Verification items for the finished model (mm, model axes). A direction names the side the tool comes from. Coordinates: 2 decimals unless noted, no trailing zeros. Write each loop counter-clockwise with the first axis right and the second up, starting at its lowest first coordinate (ties: lowest second). Pieces come first, ordered by that corner, then holes. Notation, with made-up numbers: (45.25, 66.5) -> (81.25, 66.5) arc R23 ccw to (81.25, 74.5) -> close; hole circle Ø8 at (57.25, 77.5). An arc over 180 degrees is marked (long way). Answer in a Markdown table with one row per item.
```python
from build123d import *

# Parameters (mm, degrees)
SKETCH_W        = 215
SKETCH_H        = 90
PAD_DEPTH       = 40
SKETCH001_W     = 200
SKETCH001_H     = 80
POCKET_DEPTH    = 10
SKETCH002_W     = 200
SKETCH002_H     = 13.845135
POCKET001_DEPTH = 10
POCKET002_DEPTH = 20
SKETCH004_W     = 40
SKETCH004_H     = 20
PAD001_DEPTH    = 40


with BuildPart() as part:
    # Sketch → Pad (new body)
    with BuildSketch(Plane.XY):
        Rectangle(SKETCH_W, SKETCH_H)
    extrude(amount=PAD_DEPTH)

    # Sketch001 (on Face6 of Pad) → Pocket (cut)
    with BuildSketch(Plane.XY.offset(40)):
        Rectangle(SKETCH001_W, SKETCH001_H)
    extrude(amount=-POCKET_DEPTH, mode=Mode.SUBTRACT)

    # Sketch002 (on Face5 of Pocket) → Pocket001 (cut)
    with BuildSketch(Plane.XY.offset(40)):
        with Locations((0.151818, -40.134584)):
            Rectangle(SKETCH002_W, SKETCH002_H)
    extrude(amount=-POCKET001_DEPTH, mode=Mode.SUBTRACT)

    # Sketch003 (on Face14 of Pocket001) → Pocket002 (cut)
    with BuildSketch(Plane.XY.offset(30)):
        with BuildLine():
            ThreePointArc((-50, 35), (-85, 0), (-50, -35))
            Line((-50, -35), (50, -35))
            ThreePointArc((50, -35), (85, 0), (50, 35))
            Line((50, 35), (-50, 35))
        make_face()
    extrude(amount=-POCKET002_DEPTH, mode=Mode.SUBTRACT)

    # Sketch004 (on Face6 of Pocket002) → Pad001 (join)
    with BuildSketch(Plane.XZ.offset(45)):
        with Locations((-87.5, 10)):
            Rectangle(SKETCH004_W, SKETCH004_H)
        with Locations((87.5, 10)):
            Rectangle(SKETCH004_W, SKETCH004_H)
    extrude(amount=PAD001_DEPTH)


solid = part.part
```
1. Section check C-C, the plane x = -5. Record the boundary of the cut face in (y, z).
Geometry says:
| item | result |
|---|---|
| outline | (-45, 0) -> (45, 0) -> (45, 40) -> (40, 40) -> (40, 30) -> (35, 30) -> (35, 10) -> (-35, 10) -> (-35, 30) -> (-45, 30) -> close |
2. Section check B-B, the plane z = 35. Record the boundary of the cut face in (x, y), plus the area to 3 significant figures.
Geometry says:
| item | result |
|---|---|
| outline | (-107.5, -45) -> (-99.85, -45) -> (-99.85, -40) -> (-100, -40) -> (-100, 40) -> (100, 40) -> (100, -33.21) -> (100.15, -33.21) -> (100.15, -45) -> (107.5, -45) -> (107.5, 45) -> (-107.5, 45) -> close |
| area | 2,350 mm^2 |
3. Tool access check on faces 1 (the flat face through (-1, -35, 20)), 2 (the flat face through (100.152, -39, 35)), 3 (the flat face through (87, -65, 20)), 4 (the flat face through (67.5, -65, 10)). Record the directions out of +Z, -Z, +X, -X, +Y, -Y that give a thin tool (end or side, any length) a straight path to the whole face; none if there is none.
Geometry says:
| item | result |
|---|---|
| face 1 | +Z |
| face 2 | +Z, -Y |
| face 3 | +Z, +X, -X, -Y |
| face 4 | +Z, -Z, -Y |
4. Depth check by flat-ended pin: P1, Ø6, axis at x = 11.5, z = 24.5, coming from the -Y side; P2, Ø8, axis at x = 7, z = 36, coming from the -Y side; P3, Ø4, axis at x = -48, y = -4, coming from the -Z side; P4, Ø3, axis at x = 67, y = 15, coming from the +Z side. Enter the tip coordinate at first touch or a pass-through.
Geometry says:
| item | result |
|---|---|
| P1 | y = -45 |
| P2 | y = 40 |
| P3 | z = 0 |
| P4 | z = 10 |
5. Thickness scan on line 1 (X direction, y = -46, z = 15.5); line 2 (X direction, y = -10.5, z = 37); line 3 (Y direction, x = -6, z = 25). Record the ranges inside material, lowest first. Write a range as from..to.
Geometry says:
| item | result |
|---|---|
| line 1 | -107.5..-67.5, 67.5..107.5 |
| line 2 | -107.5..-100, 100..107.5 |
| line 3 | -45..-35, 35..45 |
6. Mould release check, pull along X, two halves, no side actions. Record for faces 5 (the flat face through (-107.5, -5, 20)), 6 (the flat face through (-2, -5, 0)), 7 (the flat face through (-2, -45, 15)): released by +X, released by -X, zero draft, split by the parting line, or undercut.
Geometry says:
| item | result |
|---|---|
| face 5 | released by -X |
| face 6 | zero draft |
| face 7 | undercut |
7. Section check D-D, the plane z = 7.5. Record the boundary of the cut face in (x, y).
Geometry says:
| item | result |
|---|---|
| outline | (-107.5, -85) -> (-67.5, -85) -> (-67.5, -45) -> (67.5, -45) -> (67.5, -85) -> (107.5, -85) -> (107.5, 45) -> (-107.5, 45) -> close |
8. Section check A-A, the plane y = 0. Record the boundary of the cut face in (x, z).
Geometry says:
| item | result |
|---|---|
| outline | (-107.5, 0) -> (107.5, 0) -> (107.5, 40) -> (100, 40) -> (100, 30) -> (85, 30) -> (85, 10) -> (-85, 10) -> (-85, 30) -> (-100, 30) -> (-100, 40) -> (-107.5, 40) -> close |
